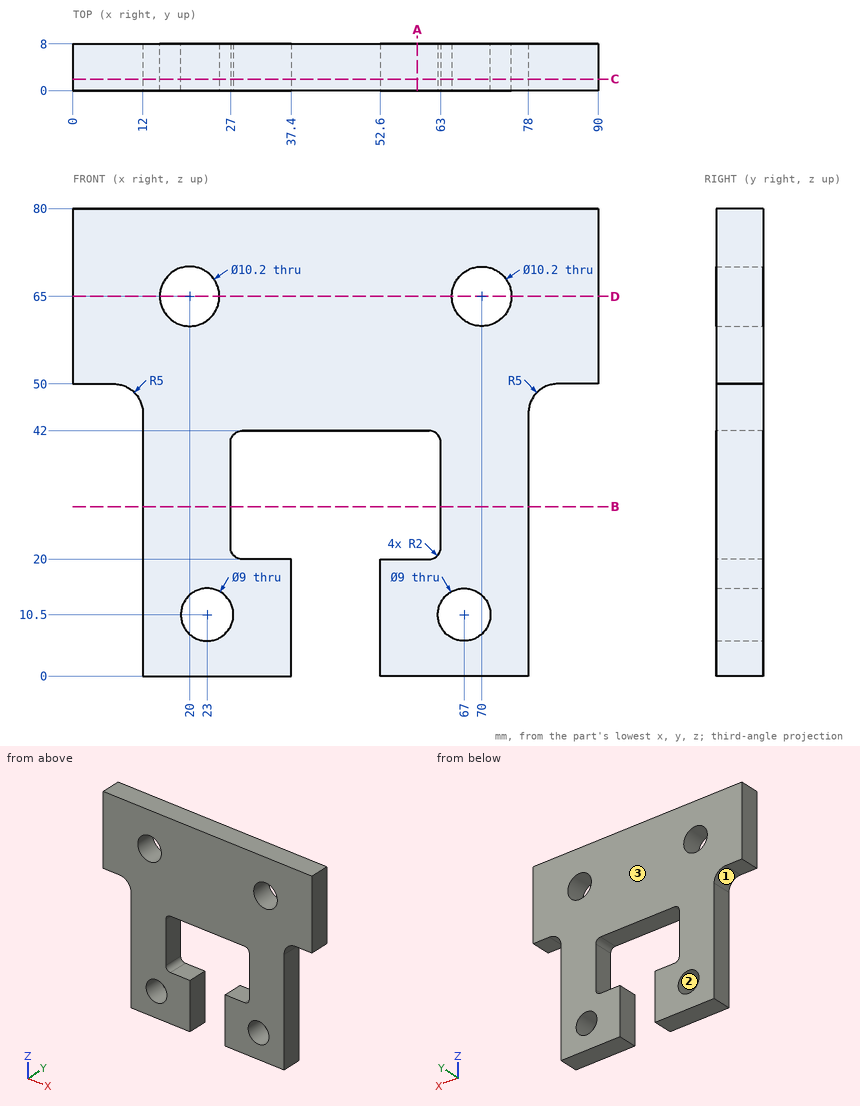
For this review, use the dimensioned drawing (mm, ordinates from the lowest corner) and the shaded views. Round coordinates to 2 decimals unless told otherwise and drop trailing zeros. Order: outer loops, then holes, each group sorted by start corner. A loop starts at its lowest first (then second) coordinate and runs counter-clockwise, first axis right, second up. Notation, with made-up numbers: M 51.25,33 L 104.25,33 A19 cw 104.25,48 Z; hole C 73.25,67.25 d1. An arc over 180 degrees is marked long. Use a Markdown table: item, result.
1) Consider section A-A (x = 59). Write out the cut boundary in (y, z), then the cut area to 3 significant figures.
Report:
| item | result |
|---|---|
| outline | M 0,0 L 8,0 L 8,20 L 0,20 Z; M 0,42 L 8,42 L 8,80 L 0,80 Z |
| area | 464 mm^2 |
2) Wall thickness on line 1 along X through (y, z) = (1.75, 22.5); line 2 along Z through (x, y) = (70, 3.25); line 3 along Z through (x, y) = (68, 2.75): over which ranges is each line inside the solid? List them lowest first. Write a range as [from, to].
Report:
| item | result |
|---|---|
| line 1 | [12, 27], [63, 78] |
| line 2 | [0, 7.15], [13.85, 59.9], [70.1, 80] |
| line 3 | [0, 6.11], [14.89, 60.31], [69.69, 80] |
3) Draft analysis for pull direction Z (two halves, no side actions). For the marked faces 1, 2 and 3, state which applies: released by +Z, released by -Z, zero draft, split by the parting line, or undercut.
Report:
| item | result |
|---|---|
| face 1 | released by -Z |
| face 2 | undercut |
| face 3 | zero draft |
4) Consider section B-B (z = 29). Write out the cut boundary in (x, y), then the cut area to 3 significant figures.
Report:
| item | result |
|---|---|
| outline | M 12,0 L 27,0 L 27,8 L 12,8 Z; M 63,0 L 78,0 L 78,8 L 63,8 Z |
| area | 240 mm^2 |
5) Consider section C-C (y = 2). Write out the cut boundary in (x, z), then the cut area to 3 significant figures.
Report:
| item | result |
|---|---|
| outline | M 0,50 L 7,50 A5 cw 12,45 L 12,0 L 37.4,0 L 37.4,20 L 29,20 A2 cw 27,22 L 27,40 A2 cw 29,42 L 61,42 A2 cw 63,40 L 63,22 A2 cw 61,20 L 52.6,20 L 52.6,0 L 78,0 L 78,45 A5 cw 83,50 L 90,50 L 90,80 L 0,80 Z; hole C 20,65 d10.2; hole C 23,10.5 d9; hole C 67,10.5 d9; hole C 70,65 d10.2 |
| area | 4,630 mm^2 |
6) Insertion check: pin 1 (4 mm diameter, centred on y = 3, z = 12, fed in from -X); pin 2 (2 mm diameter, centred on x = 3, y = 3, fed in from -Z); pin 3 (4 mm diameter, centred on y = 4, z = 5.5, fed in from +X). Each pin has a flat end and moves straight along its axis. Give the tip position at first contact, or say it passes through.
Report:
| item | result |
|---|---|
| pin 1 | x = 12 |
| pin 2 | z = 50 |
| pin 3 | x = 78 |
7) Consider section D-D (z = 65). Write out the cut boundary in (x, y).
Report:
| item | result |
|---|---|
| outline | M 0,0 L 14.9,0 L 14.9,8 L 0,8 Z; M 25.1,0 L 64.9,0 L 64.9,8 L 25.1,8 Z; M 75.1,0 L 90,0 L 90,8 L 75.1,8 Z |
